Autodesk Inventor part; units mm, degrees
sketch "Sketch1" plane through (0, 0, 0) normal (1, 0, 0) x (0, 1, 0)
  line L0 (0, 0) -> (25, 0)
  line L1 (25, 0) -> (25, -60)
  line L2 (25, -60) -> (0, -60)
  line L3 (0, -60) -> (0, 0)
  line L4 (0, -20) -> (-20, -20)
  line L5 (-20, -20) -> (-20, -40)
  line L6 (-20, -40) -> (0, -40)
  line L7 (0, -40) -> (0, -20)
  line L8 (0, 0) -> (-20, -20)
  line L9 (-20, -40) -> (0, -60)
  line L10 (0, -30) -> (-20, -30)
  circle A0 centre (-10, -30) radius 3
  dimension "d0" = 25
  dimension "d1" = 60
  dimension "d2" = 20
  dimension "d3" = 20
  dimension "d4" = 6
extrude "Extrusion1" add sketch "Sketch1" along normal blind 4 contours L0 L1 L2 L3 | L3 L4 L8 | L3 L10 A0 L5 L4 | L3 L6 L5 L10 A0 | L9 L6 L3
properties part number "stickplate"
Geometry: final body of the model. Coordinates: model frame, mm. Give positions to 0.01 mm unless a question says otherwise; leave off trailing zeros. Order: outer loops, then holes, each group sorted by start corner. A loop starts at its lowest first (then second) coordinate and runs counter-clockwise, first axis right, second up. Notation, with made-up numbers: (72, 33) -> (81, 33) arc R17 ccw to (81, 56) -> close; hole circle Ø10 at (-4.75, 46). An arc over 180 degrees is marked (long way). Write each question's results on one line, items separated by ' | '. Start each with the question number.
1) Draft query along Y for faces 1 (the flat face through (2, 13, -60)), 2 (the flat face through (2, 25, -30)), 3 (the cylindrical face through (1.97, -12.21, -32.03)). Return one class per face: pulls with the +Y half, pulls with the -Y half, needs draft (parallel to the pull), parting line crosses it, or undercut.
2) Section C-C (x = 2.05). Return loops of the section in (y, z).
3) Section B-B (z = -30). Return loops of the section in (x, y), then the cut area to 3 significant figures.
4) Section A-A (y = -10). Return loops of the section in (x, z), then the cut area to 3 significant figures.
5) First-contact query: pin 1 (2 mm diameter, centred on x = 3.5, y = -14, fed in from -Z); pin 2 (2 mm diameter, centred on x = 3, z = -53, fed in from -Y). Flat tips, straight axial feed; report the tip coordinate or a pass-through.
6) Line query: line 1 (Y direction, x = 2.65, z = -30); line 2 (Z direction, x = 1.45, y = -10); line 3 (Y direction, x = 1.1, z = -13). Output: solid intervals per line, ascending. Write a range as from..to.
7) Section D-D (y = -4.5). Return loops of the section in (x, z), then the cut area to 3 significant figures.
Calculated:
1) face 1: needs draft | face 2: pulls with the +Y half | face 3: undercut
2) outline: (-20, -40) -> (0, -60) -> (25, -60) -> (25, 0) -> (0, 0) -> (-20, -20) -> close; hole circle Ø6 at (-10, -30)
3) outline: (0, -20) -> (4, -20) -> (4, -13) -> (0, -13) -> close; (0, -7) -> (4, -7) -> (4, 25) -> (0, 25) -> close | area: 156 mm2
4) outline: (0, -50) -> (4, -50) -> (4, -33) -> (0, -33) -> close; (0, -27) -> (4, -27) -> (4, -10) -> (0, -10) -> close | area: 136 mm2
5) pin 1: z = -47 | pin 2: y = -8
6) line 1: -20..-13, -7..25 | line 2: -50..-33, -27..-10 | line 3: -13..25
7) outline: (0, -55.5) -> (4, -55.5) -> (4, -4.5) -> (0, -4.5) -> close | area: 204 mm2
